For this review, take the finished solid that the model builds, in its own axes (mm). A direction names the side the tool comes from. Coordinates: 2 decimals unless noted, no trailing zeros. Loops run counter-clockwise (first coordinate to the right, second up) from the corner with the lowest first, then second, coordinate; pieces in that order, holes last. Notation, with made-up numbers: (-29, 42.5) - (-19, 42.5) arc R21 ccw to (-19, 58.5) - close; hole circle Ø11 at (-30.75, -34). An arc over 180 degrees is marked (long way). Use one line per item in the form item = value. Start each with the question number.
1. Add section A-A on x = -3. Give the boundary of the cut face in (y, z).
2. Draft analysis for pull direction Z (two halves, no side actions). For faces 1 (the face through (-3, 6, -14.6)), 2 (the face through (-4, 6, 0)), 3 (the face through (-4, 7, -1)), 4 (the face through (-3, 0, 3)), state which applies: +Z half, -Z half, draft (parallel to the pull), parting line (faces both ways), or undercut.
3. Add section D-D on y = 8.25. Give the boundary of the cut face in (x, z).
4. Machinability: for faces 5 (the face through (-3, -1.5, -4)), 6 (the face through (-3, 0.75, -2)), 7 (the face through (0, 6, 3)), which of the approach directions +Z, -Z, +X, -X, +Y, -Y give a long, thin tool a straight path to every point of the face, cutting with its end or side? Answer none if there is none.
5. For pin 1 Ø1.8 at (x, y) = (-4, 8) entering from +Z; pin 2 Ø1.6 at (y, z) = (5.5, -2) entering from -X, all flat-tipped, find the tip position at first contact; note any pin that passes through.
6. Add section C-C on x = -6.25. Give the boundary of the cut face in (y, z).
7. To check wall thickness, follow probe 1 along Y at (x, z) = (-3, -0.3); probe 2 along Y at (x, z) = (-4, 0.25); probe 3 along Y at (x, z) = (-0.75, -1.5). State the ranges of each line that lie inside material, in increasing order.
8. Add section B-B on y = 6.6. Give the boundary of the cut face in (x, z), and give its area (3 significant figures).
```python
from build123d import *

# Parameters (mm, degrees)
F0_W     = 8
F0_H     = 16
F0_W_2   = 6
F0_H_2   = 13
F1_DEPTH = 6.6
F2_W     = 8
F2_H     = 16
F3_DEPTH = 14.6
F5_R     = 0.5
F6_DEPTH = 3
F4_W     = 12
F4_H     = 2
F7_DEPTH = 12


with BuildPart() as f1:
    # F0 (on Top) → F1 (new body)
    with BuildSketch(Plane.XY):
        with Locations((-3, 6.5)):
            Rectangle(F0_W, F0_H)
        with Locations((-3, 6.5)):
            Rectangle(F0_W_2, F0_H_2, mode=Mode.SUBTRACT)
    extrude(amount=F1_DEPTH)

    # F2 (on face) → F3 (join)
    with BuildSketch(Plane(origin=(0, 0, 0), x_dir=(1, 0, 0), z_dir=(0, 0, -1))):
        with Locations((-3, -6.5)):
            Rectangle(F2_W, F2_H)
    extrude(amount=F3_DEPTH)

    # F5 (on face) → F6 (cut)
    with BuildSketch(Plane.XY):
        with Locations((-3, 11.32)):
            Circle(F5_R)
        with Locations((-3, 6.6)):
            Circle(F5_R)
        with Locations((-3, 1.68)):
            Circle(F5_R)
    extrude(amount=-F6_DEPTH, mode=Mode.SUBTRACT)

    # F4 (on Right) → F7 (cut)
    with BuildSketch(Plane.YZ):
        with Locations((6.75, -2)):
            Rectangle(F4_W, F4_H)
    extrude(amount=-F7_DEPTH, mode=Mode.SUBTRACT)


solid = f1.part
```
Conclusion:
q1.outline = (-1.5, -14.6) - (14.5, -14.6) - (14.5, 6.6) - (13, 6.6) - (13, 0) - (11.82, 0) - (11.82, -1) - (12.75, -1) - (12.75, -3) - (0.75, -3) - (0.75, -1) - (1.18, -1) - (1.18, 0) - (0, 0) - (0, 6.6) - (-1.5, 6.6) - close; (2.18, -1) - (6.1, -1) - (6.1, 0) - (2.18, 0) - close; (7.1, -1) - (10.82, -1) - (10.82, 0) - (7.1, 0) - close
q2.face_1 = -Z half
q2.face_2 = +Z half
q2.face_3 = undercut
q2.face_4 = draft
q3.outline = (-7, -14.6) - (1, -14.6) - (1, 6.6) - (0, 6.6) - (0, 0) - (-6, 0) - (-6, 6.6) - (-7, 6.6) - (-7, -1) - (0, -1) - (0, -3) - (-7, -3) - close
q4.face_5 = +Z, -Z, +X, -X, -Y
q4.face_6 = -X
q4.face_7 = +Z
q5.pin_1 = 0
q5.pin_2 = 0
q6.outline = (-1.5, -14.6) - (14.5, -14.6) - (14.5, 6.6) - (-1.5, 6.6) - close; hole (0.75, -3) - (12.75, -3) - (12.75, -1) - (0.75, -1) - close
q7.probe_1 = -1.5 to 1.18, 2.18 to 6.1, 7.1 to 10.82, 11.82 to 14.5
q7.probe_2 = -1.5 to 0, 13 to 14.5
q7.probe_3 = -1.5 to 0.75, 12.75 to 14.5
q8.outline = (-7, -14.6) - (1, -14.6) - (1, 6.6) - (0, 6.6) - (0, 0) - (-2.5, 0) - (-2.5, -1) - (0, -1) - (0, -3) - (-7, -3) - close; (-7, -1) - (-3.5, -1) - (-3.5, 0) - (-6, 0) - (-6, 6.6) - (-7, 6.6) - close
q8.area = 115 mm^2
